from build123d import *

# Parameters (mm, degrees)
F0_R     = 12
F0_R_2   = 9
F1_DEPTH = 62
F2_R     = 12
F3_DEPTH = 2
F4_R     = 10.75
F5_DEPTH = 8


with BuildPart() as f1:
    # F0 (on Front) → F1 (new body)
    with BuildSketch(Plane.XZ):
        Circle(F0_R)
        Circle(F0_R_2, mode=Mode.SUBTRACT)
    extrude(amount=F1_DEPTH)

    # F2 (on face) → F3 (join)
    with BuildSketch(Plane(origin=(0, 0, 0), x_dir=(-1, 0, 0), z_dir=(0, 1, 0))):
        Circle(F2_R)
    extrude(amount=F3_DEPTH)

    # F4 (on face) → F5 (cut)
    with BuildSketch(Plane.XZ.offset(62)):
        Circle(F4_R)
    extrude(amount=-F5_DEPTH, mode=Mode.SUBTRACT)


solid = f1.part
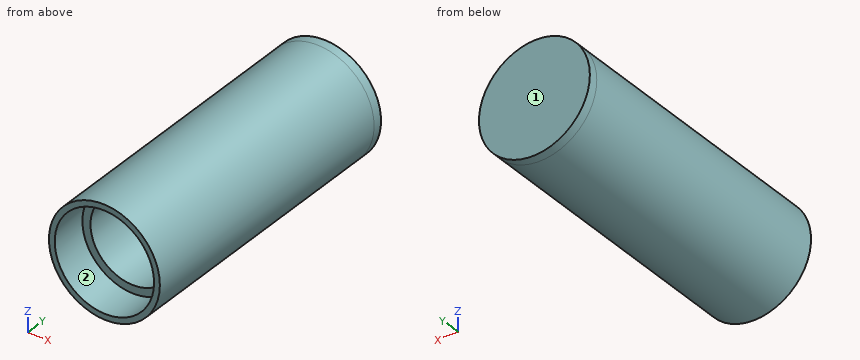
Here's how the part is built. I have some questions about the finished solid (model axes, mm). Face numbers are marked on the shaded views. Give positions to 0.01 mm unless a question says otherwise; leave off trailing zeros. Order: outer loops, then holes, each group sorted by start corner. A loop starts at its lowest first (then second) coordinate and runs counter-clockwise, first axis right, second up. Notation, with made-up numbers: (7, 43) -> (33, 43) arc R11 ccw to (33, 64) -> close; hole circle Ø1 at (-28.75, -19.75). An arc over 180 degrees is marked (long way). Use a Markdown table: item, result. Add a question column.
Item 1: I need wall thicknesses on line 1 (Z direction, x = 0, y = -15.5); line 2 (Y direction, x = -7.5, z = -3). Which ranges of each line are inside material? Lowest first, please.
Item 2: Imagine slicing it at C-C on y = -7.5. Please give me the cut outline in (x, z).
Item 3: Will these pins go through, and if not, where does the flat tip stop? pin 1 (10 mm diameter, centred on x = 8, y = -35, fed in from +Z); pin 2 (8 mm diameter, centred on y = -13.5, z = -5, fed in from -X); pin 3 (1.5 mm diameter, centred on y = -41.5, z = -5, fed in from +X).
Item 4: If we mould it in two halves opening along Z, with no side actions, what happens to the marked faces 1 and 2? For each: pulls with the +Z half, pulls with the -Z half, needs draft (parallel to the pull), parting line crosses it, or undercut.
Item 5: Imagine slicing it at D-D on y = -58. Please give me the cut outline in (x, z).
Item 6: Imagine slicing it at A-A on x = 0. Please give me the cut outline in (y, z), plus the area to 3 significant figures.
Item 7: Imagine slicing it at B-B on z = 0. Please give me the cut outline in (x, y).
Data:
| question | item | result |
|---|---|---|
| 1 | line 1 | z = -12 to -9, 9 to 12 |
| 1 | line 2 | y = 0 to 2 |
| 2 | outline | circle Ø24 at (0, 0); hole circle Ø18 at (0, 0) |
| 3 | pin 1 | stops at z = 11.62 |
| 3 | pin 2 | stops at x = -11.96 |
| 3 | pin 3 | stops at x = 11.22 |
| 4 | face 1 | needs draft |
| 4 | face 2 | undercut |
| 5 | outline | circle Ø24 at (0, 0); hole circle Ø21.5 at (0, 0) |
| 6 | outline | (-62, -12) -> (2, -12) -> (2, 12) -> (-62, 12) -> (-62, 10.75) -> (-54, 10.75) -> (-54, 9) -> (0, 9) -> (0, -9) -> (-54, -9) -> (-54, -10.75) -> (-62, -10.75) -> close |
| 6 | area | 392 mm² |
| 7 | outline | (-12, -62) -> (-10.75, -62) -> (-10.75, -54) -> (-9, -54) -> (-9, 0) -> (9, 0) -> (9, -54) -> (10.75, -54) -> (10.75, -62) -> (12, -62) -> (12, 2) -> (-12, 2) -> close |
